```python
from build123d import *

# Parameters (mm, degrees)
CEK_DONMUS_KUTU_U_1_0_1_DEPTH = 700


with BuildPart() as part:
    # Sketch1 → CEK_donmus_kutu_U_1.0_1 (new body)
    with BuildSketch(Plane.XY):
        Polygon((13.7, 82), (13.7, 8), (604.3, 8), (604.3, 82), (603.3, 82), (603.3, 9), (14.7, 9), (14.7, 82), align=None)
    extrude(amount=-CEK_DONMUS_KUTU_U_1_0_1_DEPTH)


solid = part.part
```
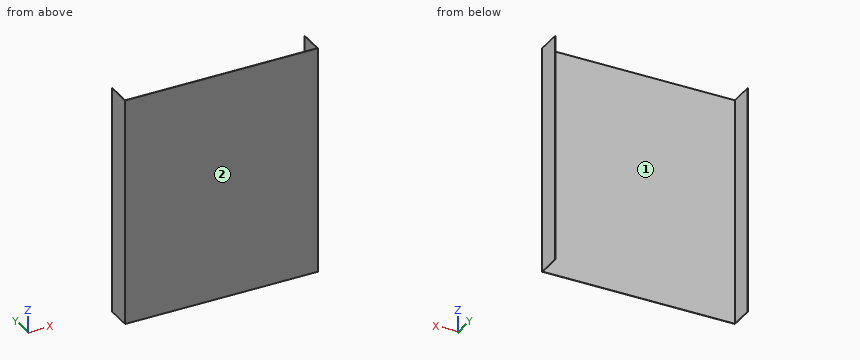
Could you check a few things on this model? Use its own coordinates, in mm. Face numbers are marked on the shaded views. Coordinates: 2 decimals unless noted, no trailing zeros. Write each loop counter-clockwise with the first axis right and the second up, starting at its lowest first coordinate (ties: lowest second). Pieces come first, ordered by that corner, then holes. Notation, with made-up numbers: (29, 18) -> (38, 18) arc R14 cw to (38, 28) -> close; hole circle Ø3 at (67, -23.75). An arc over 180 degrees is marked (long way). Write item = value, one per line. Start each with the question number.
(1) We'd pull the mould along X, two halves only. Please class the marked faces 1 and 2: released by +X, released by -X, zero draft, split by the parting line, or undercut.
(2) I want a section at B-B (z = -369). Please give me the cut outline in (x, y).
(3) I want a section at A-A (y = 19). Please give me the cut outline in (x, z), plus the area to 3 significant figures.
(4) I need wall thicknesses on line 1 (X direction, y = 18.5, z = -433.5); line 2 (Y direction, x = 363, z = -490). Which ranges of each line are inside material? Lowest first, please. Write a range as [from, to].
(5) I want a section at C-C (x = 169). Please give me the cut outline in (y, z).
Result set:
q1.face_1 = undercut
q1.face_2 = zero draft
q2.outline = (13.7, 8) -> (604.3, 8) -> (604.3, 82) -> (603.3, 82) -> (603.3, 9) -> (14.7, 9) -> (14.7, 82) -> (13.7, 82) -> close
q3.outline = (13.7, -700) -> (14.7, -700) -> (14.7, 0) -> (13.7, 0) -> close; (603.3, -700) -> (604.3, -700) -> (604.3, 0) -> (603.3, 0) -> close
q3.area = 1,400 mm2
q4.line_1 = [13.7, 14.7], [603.3, 604.3]
q4.line_2 = [8, 9]
q5.outline = (8, -700) -> (9, -700) -> (9, 0) -> (8, 0) -> close
